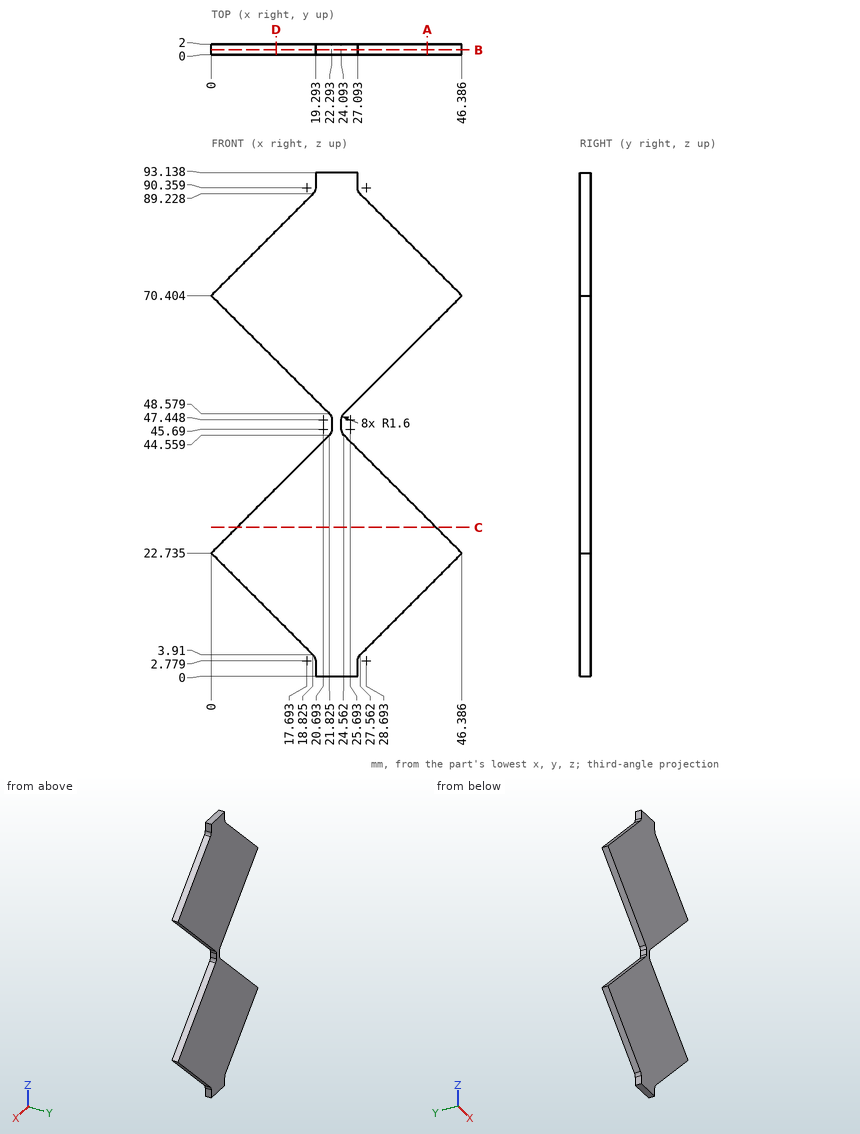
Print and shaded views of the part. All mm, measured from the part's lowest x, y and z. Round coordinates to 2 decimals unless told otherwise and drop trailing zeros. Order: outer loops, then holes, each group sorted by start corner. A loop starts at its lowest first (then second) coordinate and runs counter-clockwise, first axis right, second up.
Q1. Wall check: L1, parallel to Z at x = 19, y = 1.75 (1 decimal); L2, parallel to Z at x = 6, y = 1.35 (1 decimal); L3, parallel to X at y = 0.35, z = 25 (1 decimal). Give the ranges that are in metal, low to high.
Q2. Slice it at B-B (y = 0.9). Write the cut outline in (x, z) (1 decimal).
Q3. Drop flat-ended pins along their axis: pin 1 (0.9 mm diameter, centred on y = 1, z = 47, fed in from +X); pin 2 (0.6 mm diameter, centred on y = 1, z = 1.5, fed in from -X). Give the stop position or say it passes through.
Q4. Slice it at D-D (x = 12). Write the cut outline in (y, z) (1 decimal).
Q5. Slice it at A-A (x = 40). Write the cut outline in (y, z).
Q6. Slice it at C-C (z = 27.5). Write the cut outline in (x, y) (1 decimal).
Results below:
1. L1: z = 3.7 to 41.7, 51.4 to 89.4
1. L2: z = 16.7 to 28.7, 64.4 to 76.4
1. L3: x = 2.3 to 44.1
2. outline: (0, 22.7) - (18.8, 3.9) arc R1.6 cw to (19.3, 2.8) - (19.3, 0) - (27.1, 0) - (27.1, 2.8) arc R1.6 cw to (27.6, 3.9) - (46.4, 22.7) - (24.6, 44.6) arc R1.6 cw to (24.1, 45.7) - (24.1, 47.4) arc R1.6 cw to (24.6, 48.6) - (46.4, 70.4) - (27.6, 89.2) arc R1.6 cw to (27.1, 90.4) - (27.1, 93.1) - (19.3, 93.1) - (19.3, 90.4) arc R1.6 cw to (18.8, 89.2) - (0, 70.4) - (21.8, 48.6) arc R1.6 cw to (22.3, 47.4) - (22.3, 45.7) arc R1.6 cw to (21.8, 44.6) - close
3. pin 1: stops at x = 24.09
3. pin 2: stops at x = 19.29
4. outline: (0, 10.7) - (2, 10.7) - (2, 34.7) - (0, 34.7) - close; (0, 58.4) - (2, 58.4) - (2, 82.4) - (0, 82.4) - close
5. outline: (0, 16.35) - (2, 16.35) - (2, 29.12) - (0, 29.12) - close; (0, 64.02) - (2, 64.02) - (2, 76.79) - (0, 76.79) - close
6. outline: (4.8, 0) - (41.6, 0) - (41.6, 2) - (4.8, 2) - close
